Geometry check sheet. Reference: the model listing, model coordinates, mm. A direction names the side the tool comes from. Round coordinates to 2 decimals unless told otherwise and drop trailing zeros. Order: outer loops, then holes, each group sorted by start corner. A loop starts at its lowest first (then second) coordinate and runs counter-clockwise, first axis right, second up.
(1) Thickness scan on L1, parallel to Z at x = -20, y = -2.1; L2, parallel to X at y = -4.25, z = 100.5; L3, parallel to Z at x = -134, y = -12.5. Record the ranges inside material, lowest first.
(2) Cross-section at B-B on z = 60. Enter the section's corners in (x, y), and give its area (3 significant figures).
(3) Set-up check for faces 1 (the face through (12.196, -7.605, -2.789)), 2 (the face through (-180.132, -9, 72)): record each of +Z, -Z, +X, -X, +Y, -Y from which the full face is reachable in a straight line by a thin tool's end or side.
(4) Cross-section at D-D on z = 106.5. Enter the section's corners in (x, y), and give its area (3 significant figures).
(5) Draft check along X on faces 3 (the face through (-178.328, -9.33, 115.527)), 4 (the face through (12.196, -7.605, 143.789)), 5 (the face through (-184.289, -7.605, 143.696)). Enter one of: pulls with the +X half, pulls with the -X half, needs draft (parallel to the pull), parting line crosses it, or undercut.
(6) Gauge pin test, flat end, axial feed: P1, Ø20, axis at x = -20, z = 51.5, coming from the -Y side. Record the tip position at first contact, or that the pin passes through.
(7) Cross-section at C-C on x = -118. Enter the section's corners in (y, z).
(8) Cross-section at A-A on x = -20. Enter the section's corners in (y, z), and give its area (3 significant figures).
from build123d import *

# Parameters (mm, degrees)
F0_W     = 14
F0_H     = 23.5
F0_R     = 2.5
F1_DEPTH = 15
F2_DEPTH = 3.5
F3_R     = 6
F4_R     = 11
F5_DEPTH = 25


with BuildPart() as f1:
    # F0 (on Front) → F1 (new body)
    with BuildSketch(Plane.XZ):
        with Locations((-179, 133.75)):
            Rectangle(F0_W, F0_H)
        with Locations((-181.5, 141)):
            Circle(F0_R, mode=Mode.SUBTRACT)
        Polygon((0, 145.5), (-172, 145.5), (-172, 122), (-186, 122), (-186, 19), (-172, 19), (-172, -4.5), (0, -4.5), (0, 19), (14, 19), (14, 122), (0, 122), align=None)
        Polygon((-167.763814, 139.657289), (-5.603518, 139.657289), (-5.603518, 117.238402), (10.543795, 117.238402), (10.543795, 26.938597), (-5.603518, 26.938597), (-5.603518, 0), (-167.763814, 0), (-167.763814, 26.938597), (-180.131972, 26.938597), (-180.131972, 117.238402), (-167.763814, 117.238402), align=None, mode=Mode.SUBTRACT)
        with Locations((7, 133.75)):
            Rectangle(F0_W, F0_H)
        with Locations((9.5, 141)):
            Circle(F0_R, mode=Mode.SUBTRACT)
        with Locations((-179, 7.25)):
            Rectangle(F0_W, F0_H)
        with Locations((-181.5, 0)):
            Circle(F0_R, mode=Mode.SUBTRACT)
        with Locations((7, 7.25)):
            Rectangle(F0_W, F0_H)
        with Locations((9.5, 0)):
            Circle(F0_R, mode=Mode.SUBTRACT)
    extrude(amount=F1_DEPTH)

    # F0 (on Front) → F2 (join)
    with BuildSketch(Plane.XZ):
        Polygon((-5.603518, 117.238402), (-5.603518, 139.657289), (-167.763814, 139.657289), (-167.763814, 117.238402), (-180.131972, 117.238402), (-180.131972, 26.938597), (-167.763814, 26.938597), (-167.763814, 0), (-5.603518, 0), (-5.603518, 26.938597), (10.543795, 26.938597), (10.543795, 117.238402), align=None)
    extrude(amount=F2_DEPTH)

    # F3
    f3_edges = [f1.edges().sort_by_distance(p)[0] for p in [
        (-186, -7.5, 145.5),
        (-186, -7.5, -4.5),
        (14, -7.5, -4.5),
        (14, -7.5, 145.5),
        (-180.131972, -9.25, 26.938597),
        (-167.763814, -9.25, 26.938597),
        (-167.763814, -9.25, 0),
        (-5.603518, -9.25, 0),
        (-5.603518, -9.25, 26.938597),
        (10.543795, -9.25, 26.938597),
        (-180.131972, -9.25, 117.238402),
        (-167.763814, -9.25, 117.238402),
        (-167.763814, -9.25, 139.657289),
        (10.543795, -9.25, 117.238402),
        (-5.603518, -9.25, 117.238402),
        (-5.603518, -9.25, 139.657289),
    ]]
    fillet(f3_edges, radius=F3_R)

    # F4 (on face) → F5 (cut)
    with BuildSketch(Plane.XZ.offset(3.5)):
        with Locations((-20, 124.5)):
            Circle(F4_R)
        with Locations((-20, 90.5)):
            Circle(F4_R)
        with Locations((-20, 51.5)):
            Circle(F4_R)
        with Locations((-20, 17.5)):
            Circle(F4_R)
    extrude(amount=-F5_DEPTH, mode=Mode.SUBTRACT)


solid = f1.part
Found:
1. L1: z = -4.5 to 6.5, 28.5 to 40.5, 62.5 to 79.5, 101.5 to 113.5, 135.5 to 145.5
1. L2: x = -186 to -180.13, 10.54 to 14
1. L3: z = -4.5 to 0, 139.66 to 145.5
2. outline: (-186, -15) - (-180.13, -15) - (-180.13, -3.5) - (-26.98, -3.5) - (-26.98, 0) - (-186, 0) - close; (-13.02, -3.5) - (10.54, -3.5) - (10.54, -15) - (14, -15) - (14, 0) - (-13.02, 0) - close
2. area: 758 mm2
3. face 1: -Z, +X, +Y, -Y
3. face 2: -Y
4. outline: (-186, -15) - (-180.13, -15) - (-180.13, -3.5) - (10.54, -3.5) - (10.54, -15) - (14, -15) - (14, 0) - (-186, 0) - close
4. area: 807 mm2
5. face 3: undercut
5. face 4: pulls with the +X half
5. face 5: pulls with the -X half
6. P1: passes through
7. outline: (-15, -4.5) - (0, -4.5) - (0, 145.5) - (-15, 145.5) - (-15, 139.66) - (-3.5, 139.66) - (-3.5, 0) - (-15, 0) - close
8. outline: (-15, -4.5) - (0, -4.5) - (0, 6.5) - (-3.5, 6.5) - (-3.5, 0) - (-15, 0) - close; (-15, 139.66) - (-3.5, 139.66) - (-3.5, 135.5) - (0, 135.5) - (0, 145.5) - (-15, 145.5) - close; (-3.5, 28.5) - (0, 28.5) - (0, 40.5) - (-3.5, 40.5) - close; (-3.5, 62.5) - (0, 62.5) - (0, 79.5) - (-3.5, 79.5) - close; (-3.5, 101.5) - (0, 101.5) - (0, 113.5) - (-3.5, 113.5) - close
8. area: 336 mm2
